Input: dimensioned drawing with shaded views. Units: mm. Origin: part minimum x, y, z. A direction names the side the tool comes from. Round coordinates to 2 decimals unless told otherwise and drop trailing zeros. Write each loop counter-clockwise with the first axis right and the second up, starting at its lowest first coordinate (ties: lowest second). Pieces come first, ordered by that corner, then holes. Notation, with made-up numbers: M 72,65 L 115,65 A10 cw 115,78 Z; hole C -17,52 d11. An arc over 180 degrees is marked long. Answer as CSV lines item,"result". Start each with the question number.
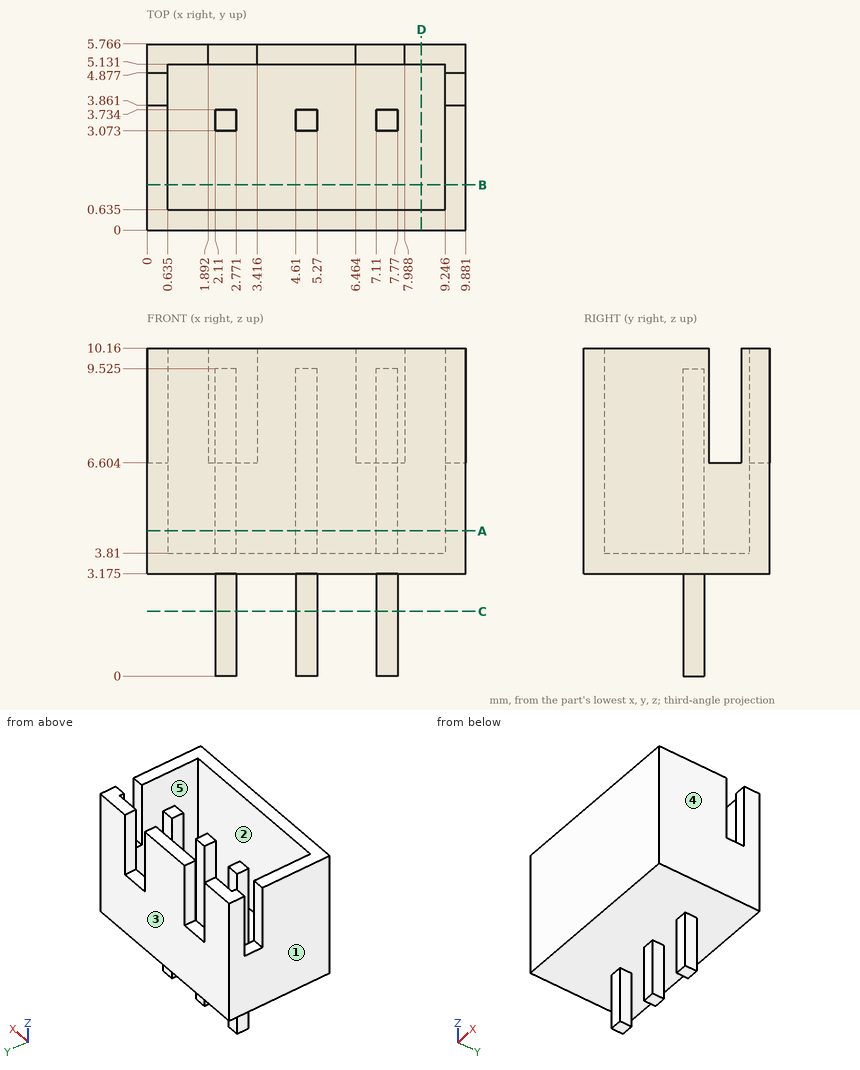
Item 1: Line query: line 1 (X direction, y = 3.2, z = 7) (1 decimal); line 2 (Y direction, x = 5.5, z = 4) (1 decimal); line 3 (X direction, y = 0.8, z = 5.25) (1 decimal). Output: solid intervals per line, ascending. Write a range as [from, to].
Item 2: Draft query along X for the marked faces 1, 2 and 3. Return one class per face: +X half, -X half, draft (parallel to the pull), parting line (faces both ways), or undercut.
Item 3: Cut plane C-C, the plane z = 2. Return loops of the section in (x, y).
Item 4: Access query for the marked faces 4 and 5. Directions: +Z, -Z, +X, -X, +Y, -Y. A direction counts if a zero-diameter tool reaches every point of the face in a straight line with its end or side. Return the directions, or none.
Item 5: Cut plane B-B, the plane y = 1.4. Return loops of the section in (x, z) (1 decimal).
Item 6: Pin query (flat end, axial travel): pin 1 Ø0.5 at (x, z) = (9.5, 9) entering from -Y; pin 2 Ø0.7 at (y, z) = (3.5, 2) entering from -X; pin 3 Ø0.7 at (x, z) = (7.5, 1) entering from -Y. Return the tip coordinate at first contact, or that it passes through.
Item 7: Cut plane D-D, the plane x = 8.5. Return loops of the section in (y, z) (1 decimal).
Item 8: Cut plane A-A, the plane z = 4.5. Return loops of the section in (x, y) (1 decimal).
Results list:
1,line 1,"[0, 0.6], [2.1, 2.8], [4.6, 5.3], [7.1, 7.8], [9.2, 9.9]"
1,line 2,"[0, 0.6], [5.1, 5.8]"
1,line 3,"[0, 0.6], [9.2, 9.9]"
2,face 1,"-X half"
2,face 2,"undercut"
2,face 3,"draft"
3,outline,"M 2.11,3.07 L 2.77,3.07 L 2.77,3.73 L 2.11,3.73 Z; M 4.61,3.07 L 5.27,3.07 L 5.27,3.73 L 4.61,3.73 Z; M 7.11,3.07 L 7.77,3.07 L 7.77,3.73 L 7.11,3.73 Z"
4,face 4,"+Z, -Z, +X, +Y, -Y"
4,face 5,"+Z"
5,outline,"M 0,3.2 L 9.9,3.2 L 9.9,10.2 L 9.2,10.2 L 9.2,3.8 L 0.6,3.8 L 0.6,10.2 L 0,10.2 Z"
6,pin 1,"y = 0"
6,pin 2,"x = 2.11"
6,pin 3,"y = 3.07"
7,outline,"M 0,3.2 L 5.8,3.2 L 5.8,10.2 L 5.1,10.2 L 5.1,3.8 L 0.6,3.8 L 0.6,10.2 L 0,10.2 Z"
8,outline,"M 0,0 L 9.9,0 L 9.9,5.8 L 0,5.8 Z; M 2.1,3.1 L 2.8,3.1 L 2.8,3.7 L 2.1,3.7 Z; M 4.6,3.1 L 5.3,3.1 L 5.3,3.7 L 4.6,3.7 Z; M 7.1,3.1 L 7.8,3.1 L 7.8,3.7 L 7.1,3.7 Z; hole M 0.6,0.6 L 9.2,0.6 L 9.2,5.1 L 0.6,5.1 Z"
